from build123d import *

# Parameters (mm, degrees)
CROQUIS1_W              = 27.5
CROQUIS1_H              = 5.5
CROQUIS1_R              = 0.625
SALIENTE_EXTRUIR1_DEPTH = 2
REDONDEO1_R             = 1


with BuildPart() as part:
    # Croquis1 → Saliente-Extruir1 (new body)
    with BuildSketch(Plane(origin=(0, 0, 0), x_dir=(1, 0, 0), z_dir=(0, 1, 0))):
        Rectangle(CROQUIS1_W, CROQUIS1_H)
        with Locations(Location((-10.75, 0, 0), (0, 0, 270))):
            Circle(CROQUIS1_R, mode=Mode.SUBTRACT)
        with Locations(Location((10.75, 0, 0), (0, 0, 90))):
            Circle(CROQUIS1_R, mode=Mode.SUBTRACT)
    extrude(amount=SALIENTE_EXTRUIR1_DEPTH)

    # Redondeo1
    redondeo1_edges = [part.edges().sort_by_distance(p)[0] for p in [
        (13.75, 1, 2.75),
        (-13.75, 1, 2.75),
        (-13.75, 1, -2.75),
        (13.75, 1, -2.75),
    ]]
    fillet(redondeo1_edges, radius=REDONDEO1_R)


solid = part.part
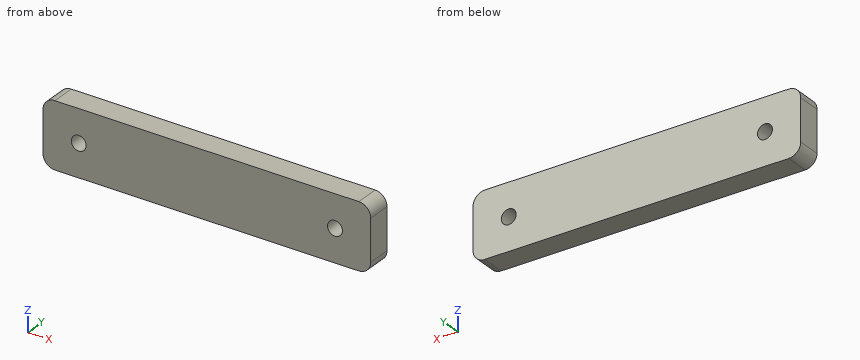
Geometry: final body of the model. Coordinates: model frame, mm. Round coordinates to 2 decimals unless told otherwise and drop trailing zeros. Loops run counter-clockwise (first coordinate to the right, second up) from the corner with the lowest first, then second, coordinate; pieces in that order, holes last. Notation, with made-up numbers: M -18,-37.75 L -6,-37.75 A20 ccw -6,-18.75 Z; hole C 43.5,78 d9. An arc over 180 degrees is marked long. Put each result on its own line as item: value. Start each with the question number.
(1) Section query A-A (z = 0). Return loops of the section in (x, y) (3 decimals), then the cut area to 3 significant figures.
(2) Material intervals for line 1 along X through (y, z) = (0.6, 0) (3 decimals); line 2 along Z through (x, y) = (10.75, 1) (3 decimals); line 3 along X through (y, z) = (1.2, 2.45), sorted ascending. Write a range as [from, to].
(3) Section query C-C (x = 10.75). Return loops of the section in (y, z) (3 decimals), then the cut area to 3 significant figures.
(4) Section query B-B (y = 1.45). Return loops of the section in (x, z) (3 decimals), then the cut area to 3 significant figures.
Findings below:
1. outline: M -13.75,0 L -11.375,0 L -11.375,2 L -13.75,2 Z; M -10.125,0 L 10.125,0 L 10.125,2 L -10.125,2 Z; M 11.375,0 L 13.75,0 L 13.75,2 L 11.375,2 Z
1. area: 50.0 mm2
2. line 1: x = [-13.75, -11.375], [-10.125, 10.125], [11.375, 13.75]
2. line 2: z = [-2.75, -0.625], [0.625, 2.75]
2. line 3: x = [-13.46, 13.46]
3. outline: M 0,-2.75 L 2,-2.75 L 2,-0.625 L 0,-0.625 Z; M 0,0.625 L 2,0.625 L 2,2.75 L 0,2.75 Z
3. area: 8.50 mm2
4. outline: M -13.75,-1.75 A1 ccw -12.75,-2.75 L 12.75,-2.75 A1 ccw 13.75,-1.75 L 13.75,1.75 A1 ccw 12.75,2.75 L -12.75,2.75 A1 ccw -13.75,1.75 Z; hole C -10.75,0 d1.25; hole C 10.75,0 d1.25
4. area: 148 mm2
